from build123d import *

# Parameters (mm, degrees)
SKETCH_2_W      = 27.85
SKETCH_2_H      = 27.85
SKETCH_2_R      = 1.25
SKETCH_2_R_2    = 11
EXTRUDE_1_DEPTH = 4
CHAMFER_1_SIZE  = 0.8


with BuildPart() as part:
    # Эскиз2 → Бобышка-Вытянуть1 (new body)
    with BuildSketch(Plane(origin=(0, 0, 0), x_dir=(1, 0, 0), z_dir=(0, 1, 0))):
        Rectangle(SKETCH_2_W, SKETCH_2_H)
        with Locations((-11.5, 11.5)):
            Circle(SKETCH_2_R, mode=Mode.SUBTRACT)
        with Locations((-11.5, -11.5)):
            Circle(SKETCH_2_R, mode=Mode.SUBTRACT)
        with Locations((11.5, -11.5)):
            Circle(SKETCH_2_R, mode=Mode.SUBTRACT)
        with Locations((11.5, 11.5)):
            Circle(SKETCH_2_R, mode=Mode.SUBTRACT)
        Circle(SKETCH_2_R_2, mode=Mode.SUBTRACT)
    extrude(amount=EXTRUDE_1_DEPTH)

    # Фаска1
    chamfer_1_edges = [part.edges().sort_by_distance(p)[0] for p in [
        (13.925, 2, -13.925),
        (13.925, 2, 13.925),
        (-13.925, 2, 13.925),
        (-13.925, 2, -13.925),
    ]]
    chamfer(chamfer_1_edges, length=CHAMFER_1_SIZE)


solid = part.part
Source: CAD feature listing. Evaluate the final solid. Frame: model axes, mm. Round coordinates to 2 decimals unless told otherwise and drop trailing zeros. Order: outer loops, then holes, each group sorted by start corner. A loop starts at its lowest first (then second) coordinate and runs counter-clockwise, first axis right, second up. Notation, with made-up numbers: (7.25, -32.75) - (52.25, -32.75) arc R20 ccw to (52.25, -22.75) - close; hole circle Ø1 at (7, -21.75). An arc over 180 degrees is marked (long way). Use a Markdown table: item, result. Add a question column.
1. Line query: probe 1 along Z at (x, y) = (-11.5, 2.2) (3 decimals); probe 2 along Z at (x, y) = (-5.75, 3) (1 decimal). Output: solid intervals per line, ascending.
2. Section query D-D (y = 1.15). Return the cut outline in (x, z) (3 decimals), then the cut area to 3 significant figures.
3. Section query C-C (x = 11.5). Return the cut outline in (y, z) (3 decimals), then the cut area to 3 significant figures.
4. Mould query, pull axis Z, two halves, no side actions, for faces 1 (the flat face through (13.53, 1.97, 13.52)), 2 (the flat face through (13.925, 2, 0)), 3 (the cylindrical face through (-2.38, 1.97, 10.74)). Classes: +Z half, -Z half, draft (parallel to the pull), parting line (faces both ways), or undercut.
5. Section query B-B (x = 0). Return the cut outline in (y, z) (3 decimals).
6. Section query A-A (z = 0). Return the cut outline in (x, y) (3 decimals), then the cut area to 3 significant figures.
Derived:
| question | item | result |
|---|---|---|
| 1 | probe 1 | -13.925 to -12.75, -10.25 to 10.25, 12.75 to 13.925 |
| 1 | probe 2 | -13.9 to -9.4, 9.4 to 13.9 |
| 2 | outline | (-13.925, -13.125) - (-13.125, -13.925) - (13.125, -13.925) - (13.925, -13.125) - (13.925, 13.125) - (13.125, 13.925) - (-13.125, 13.925) - (-13.925, 13.125) - close; hole circle Ø2.5 at (-11.5, -11.5); hole circle Ø2.5 at (-11.5, 11.5); hole circle Ø22 at (0, 0); hole circle Ø2.5 at (11.5, -11.5); hole circle Ø2.5 at (11.5, 11.5) |
| 2 | area | 375 mm2 |
| 3 | outline | (0, -13.925) - (4, -13.925) - (4, -12.75) - (0, -12.75) - close; (0, -10.25) - (4, -10.25) - (4, 10.25) - (0, 10.25) - close; (0, 12.75) - (4, 12.75) - (4, 13.925) - (0, 13.925) - close |
| 3 | area | 91.4 mm2 |
| 4 | face 1 | +Z half |
| 4 | face 2 | draft |
| 4 | face 3 | undercut |
| 5 | outline | (0, -13.925) - (4, -13.925) - (4, -11) - (0, -11) - close; (0, 11) - (4, 11) - (4, 13.925) - (0, 13.925) - close |
| 6 | outline | (-13.925, 0) - (-11, 0) - (-11, 4) - (-13.925, 4) - close; (11, 0) - (13.925, 0) - (13.925, 4) - (11, 4) - close |
| 6 | area | 23.4 mm2 |
